Design review of the part built by this model. Coordinates are the model's own, in mm. Face numbers are marked on the shaded views. A direction names the side the tool comes from. Give positions to 0.01 mm unless a question says otherwise; leave off trailing zeros. Loops run counter-clockwise (first coordinate to the right, second up) from the corner with the lowest first, then second, coordinate; pieces in that order, holes last. Notation, with made-up numbers: (82.25, 67) -> (101.25, 67) arc R27 cw to (101.25, 102) -> close; hole circle Ø1 at (39, -35.5). An arc over 180 degrees is marked (long way). Answer in a Markdown table with one row per item. Add a question column.
(1) Consider section C-C on z = 14.9. Write out the cut boundary in (x, y), then the cut area to 3 significant figures.
(2) Consider section A-A on x = -4. Write out the cut boundary in (y, z), then the cut area to 3 significant figures.
(3) For line 1 (Z direction, x = -4, y = -6); line 2 (Z direction, x = 9.9, y = 5.7); line 3 (Y direction, x = 31, z = 6.5), list the stretches that pass through material, from the lowest coordinate up.
(4) Consider section D-D on x = 25.5. Write out the cut boundary in (y, z).
(5) For the marked faces 1, 2, 3 and 4, list the 3-axis set-ups (+Z, -Z, +X, -X, +Y, -Y) from which the entire face can be reached by the end or side of a thin tool; tool diameter is ignored.
(6) Consider section B-B on y = -7. Write out the cut boundary in (x, z), then the cut area to 3 significant figures.
(7) For pin 1 (4 mm diameter, centred on x = 9.9, z = 9.9, fed in from +Y); pin 2 (6 mm diameter, centred on x = -3.5, z = 7.5, fed in from -Y); pin 3 (10 mm diameter, centred on x = 19, z = 3.5, fed in from +Y); pin 4 (10 mm diameter, centred on x = 24, z = 3, fed in from +Y), all flat-tipped, find the tip position at first contact; note any pin that passes through.
Autodesk Inventor part; units mm, degrees
ref_plane "YZ Plane" through (0, 0, 0) normal (1, 0, 0) x (0, 1, 0)
ref_plane "XZ Plane" through (0, 0, 0) normal (0, 1, 0) x (-1, 0, 0)
ref_plane "XY Plane" through (0, 0, 0) normal (0, 0, 1) x (1, 0, 0)
sketch "Эскиз1" plane through (0, 0, 0) normal (0, 0, 1) x (1, 0, 0)
  line L0 (0, 0) -> (40, 0)
  line L1 (40, 0) -> (40, -36.5)
  line L2 (40, -36.5) -> (0, -36.5)
  line L3 (0, -36.5) -> (0, 0)
  dimension "d0" = 36.5
  dimension "d1" = 40
extrude "Выдавливание1" add sketch "Эскиз1" along normal blind 19.8
sketch "Эскиз2" plane through (0, 0, 0) normal (0, 1, 0) x (1, 0, 0)
  line L0 (0, 0) -> (0, -19.8)
  line L1 (40, 0) -> (0, 0)
  circle A0 centre (9.9, -9.9) radius 9.9
  line L2 (9.9, 0) -> (34.3, 0)
  line L3 (34.3, 0) -> (34.3, -19.8)
  line L4 (34.3, -19.8) -> (9.9, -19.8)
  line L5 (9.9, -19.8) -> (9.9, 0)
  line L6 (40, 0) -> (40, -19.8)
  circle A1 centre (31.4618, -9.9) radius 5.0382
  point P0 (0, -9.9)
  point P1 (36.5, -9.9)
  point P2 (9.9, 0)
  point P3 (9.9, -19.8)
  point P4 (34.3, -14.0627)
  point P5 (34.3, -5.7373)
  dimension "d4" = 9.9
  dimension "d5" = 9.9
  dimension "d6" = 5.7
  dimension "d7" = 3.5
extrude "Выдавливание2" add sketch "Эскиз2" along normal blind 2.4 contours A0 L5 | L1 L3 A1 L4 A0 | A0 L5 | A1 L3 | L3 A1
sketch "Эскиз3" plane through (0, 2.4, 0) normal (0, 1, 0) x (1, 0, 0)
  line L0 (0, -9.9) -> (0, -19.8)
  circle A0 centre (9.9, -9.9) radius 6.6
  point P0 (0, 0)
  point P1 (9.9, 0)
  dimension "d10" = 13.2
extrude "Выдавливание3" add sketch "Эскиз3" along normal blind 1.8
sketch "Эскиз4" plane through (9.9, 4.2, 9.9) normal (0, 1, 0) x (1, 0, 0)
  circle A0 centre (0, 0) radius 2.95
  circle A1 centre (0, 0) radius 1.25
  point P0 (-9.9, 9.9)
  dimension "d13" = 5.9
  dimension "d16" = 2.5
extrude "Выдавливание4" add sketch "Эскиз4" along normal blind 3.5
sketch "Эскиз5" plane through (40, -36.5, 0) normal (1, 0, 0) x (0, 0, -1)
  line L0 (-19.8, 0) -> (-19.8, 36.5)
  line L1 (0, 0) -> (0, 36.5)
  line L2 (-19.8, 28.4) -> (0, 28.4)
  line L3 (0, 28.4) -> (0, 30.8)
  line L4 (0, 30.8) -> (-19.8, 30.8)
  line L5 (-19.8, 30.8) -> (-19.8, 28.4)
  line L6 (0, 0) -> (-19.8, 0)
  point P0 (0, 28.4)
  dimension "d17" = 28.4
  dimension "d18" = 2.4
extrude "Выдавливание5" add sketch "Эскиз5" along normal blind 7 contours L0 L4 L1 L2
sketch "Эскиз6" plane through (0, -36.5, 0) normal (-1, 0, 0) x (0, 0, 1)
  line L0 (19.8, 30.8) -> (0, 30.8)
  line L1 (0, 28.4) -> (19.8, 28.4)
  line L2 (0, 30.8) -> (19.8, 30.8)
  line L3 (19.8, 30.8) -> (19.8, 28.4)
  line L4 (19.8, 28.4) -> (0, 28.4)
  line L5 (0, 28.4) -> (0, 30.8)
  point P0 (0, 36.5)
extrude "Выдавливание6" add sketch "Эскиз6" along normal blind 7
sketch "Эскиз7" plane through (0, -5.7, 19.8) normal (0, 1, 0) x (1, 0, 0)
  line L0 (-7, 0) -> (-7, 19.8)
  circle A0 centre (-4, 14.9) radius 2
  circle A1 centre (44, 14.9) radius 2
  line L1 (47, 19.8) -> (47, 0)
  circle A2 centre (-4, 4.9) radius 2
  circle A3 centre (44, 4.9) radius 2
  point P0 (0, 19.8)
  point P1 (-7, 9.9)
  dimension "d23" = 4
  dimension "d24" = 5
  dimension "d25" = 3
  dimension "d26" = 4
  dimension "d27" = 48
  dimension "d28" = 3
  dimension "d29" = 4
  dimension "d30" = 5
extrude "Выдавливание7" cut sketch "Эскиз7" against normal blind 10
fillet "Сопряжение1" radius 1 4 edges at (-7, -6.9, 19.8) (-7, -6.9, 0) (47, -6.9, 19.8) (47, -6.9, 0)
chamfer "Фаска1" distance 2 angle 45 4 edges at (20, -36.5, 0) (0, -36.5, 9.9) (20, -36.5, 19.8) (40, -36.5, 9.9)
fillet "Сопряжение3" radius 0.5 10 edges at (0, -21.3, 0) (0, -21.3, 19.8) (0, -2.85, 0) (0, -2.85, 19.8) (40, -21.3, 0) (40, -2.85, 0) (34.3, 1.2, 0) (34.3, 1.2, 19.8) (40, -2.85, 19.8) (40, -21.3, 19.8)
sketch "Эскиз8" plane through (47, -36.5, 0) normal (1, 0, 0) x (0, 0, -1)
  line L0 (-0.5, 30.8) -> (-19.3, 30.8)
  line L1 (-19.3, 28.4) -> (-0.5, 28.4)
  line L2 (-13.9, 30.8) -> (-15.9, 30.8)
  line L3 (-15.9, 30.8) -> (-15.9, 28.4)
  line L4 (-15.9, 28.4) -> (-13.9, 28.4)
  line L5 (-13.9, 28.4) -> (-13.9, 30.8)
  line L6 (-1, 30.8) -> (-18.8, 30.8)
  line L7 (-18.8, 28.4) -> (-1, 28.4)
  line L8 (-5.9, 30.8) -> (-3.9, 30.8)
  line L9 (-3.9, 30.8) -> (-3.9, 28.4)
  line L10 (-3.9, 28.4) -> (-5.9, 28.4)
  line L11 (-5.9, 28.4) -> (-5.9, 30.8)
  point P0 (0, 36.5)
  point P1 (-9.9, 30.8)
  point P2 (-14.9, 31.074)
  point P3 (-4.9, 31.074)
  point P4 (-14.9, 30.8)
  dimension "d39" = 5
  dimension "d40" = 1
  dimension "d41" = 4
  dimension "d42" = 4
  dimension "d43" = 6
extrude "Выдавливание8" cut sketch "Эскиз8" against normal blind 2 contours L9 L1 L11 L0 | L5 L1 L3 L0
sketch "Эскиз9" plane through (-7, -36.5, 0) normal (-1, 0, 0) x (0, 0, 1)
  line L0 (18.8, 30.8) -> (1, 30.8)
  line L1 (1, 28.4) -> (18.8, 28.4)
  line L2 (5.9, 30.8) -> (3.9, 30.8)
  line L3 (3.9, 30.8) -> (3.9, 28.4)
  line L4 (3.9, 28.4) -> (5.9, 28.4)
  line L5 (5.9, 28.4) -> (5.9, 30.8)
  line L6 (13.9, 30.8) -> (15.9, 30.8)
  line L7 (15.9, 30.8) -> (15.9, 28.4)
  line L8 (15.9, 28.4) -> (13.9, 28.4)
  line L9 (13.9, 28.4) -> (13.9, 30.8)
  point P0 (0, 36.5)
  point P1 (9.9, 30.8)
  dimension "d46" = 4
  dimension "d47" = 6
  dimension "d48" = 4
  dimension "d49" = 6
extrude "Выдавливание9" cut sketch "Эскиз9" against normal blind 2 contours L7 L1 L9 L0 | L5 L1 L3 L0
properties part number "MG996R" material "Чугун, литейный"
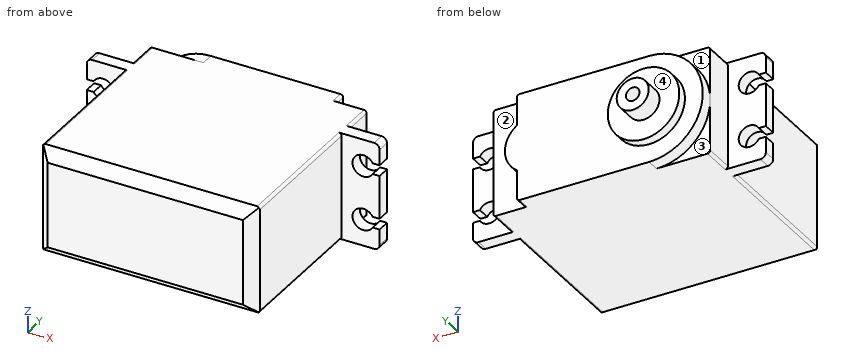
Values follow:
| question | item | result |
|---|---|---|
| 1 | outline | (-2, -8.1) -> (0, -8.1) -> (0, -34.5) -> (2, -36.5) -> (38, -36.5) -> (40, -34.5) -> (40, -8.1) -> (42, -8.1) -> (42, -5.7) -> (40, -5.7) -> (40, 0) -> (34.3, 0) -> (34.3, 2.4) -> (14.21, 2.4) -> (14.21, 4.2) -> (5.59, 4.2) -> (5.59, 2.4) -> (1.36, 2.4) -> (1.36, 0) -> (0, 0) -> (0, -5.7) -> (-2, -5.7) -> close |
| 1 | area | 1,560 mm2 |
| 2 | outline | (-8.1, 0) -> (-5.7, 0) -> (-5.7, 2.9) -> (-8.1, 2.9) -> close; (-8.1, 6.9) -> (-5.7, 6.9) -> (-5.7, 12.9) -> (-8.1, 12.9) -> close; (-8.1, 16.9) -> (-5.7, 16.9) -> (-5.7, 19.8) -> (-8.1, 19.8) -> close |
| 2 | area | 28.3 mm2 |
| 3 | line 1 | 0 to 2.9, 6.9 to 12.9, 16.9 to 19.8 |
| 3 | line 2 | 6.95 to 8.65, 11.15 to 12.85 |
| 3 | line 3 | -36.5 to 2.4 |
| 4 | outline | (-36.5, 2) -> (-34.5, 0) -> (2.4, 0) -> (2.4, 19.8) -> (-34.5, 19.8) -> (-36.5, 17.8) -> close |
| 5 | face 1 | +Z, -X, +Y |
| 5 | face 2 | +X, +Y |
| 5 | face 3 | -Z, -X, +Y |
| 5 | face 4 | +Y |
| 6 | outline | (-7, 1) arc R1 ccw to (-6, 0) -> (46, 0) arc R1 ccw to (47, 1) -> (47, 3.9) -> (45.73, 3.9) arc R2 cw (long way) to (45.73, 5.9) -> (47, 5.9) -> (47, 13.9) -> (45.73, 13.9) arc R2 cw (long way) to (45.73, 15.9) -> (47, 15.9) -> (47, 18.8) arc R1 ccw to (46, 19.8) -> (-6, 19.8) arc R1 ccw to (-7, 18.8) -> (-7, 15.9) -> (-5.73, 15.9) arc R2 cw (long way) to (-5.73, 13.9) -> (-7, 13.9) -> (-7, 5.9) -> (-5.73, 5.9) arc R2 cw (long way) to (-5.73, 3.9) -> (-7, 3.9) -> close |
| 6 | area | 1,010 mm2 |
| 7 | pin 1 | y = 7.7 |
| 7 | pin 2 | y = -8.1 |
| 7 | pin 3 | y = 4.2 |
| 7 | pin 4 | y = 2.4 |
